Check sheet for the drawn part. Datum: minimum x, y, z corner. Units: mm. A direction names the side the tool comes from. Round coordinates to 2 decimals unless told otherwise and drop trailing zeros. Loops run counter-clockwise (first coordinate to the right, second up) from the corner with the lowest first, then second, coordinate; pieces in that order, holes last. Notation, with made-up numbers: (18.5, 16.5) -> (48.5, 16.5) arc R7 ccw to (48.5, 28.5) -> close; hole circle Ø9 at (34.5, 13). An arc over 180 degrees is marked (long way). Write item = value, one per line. Start each with the question number.
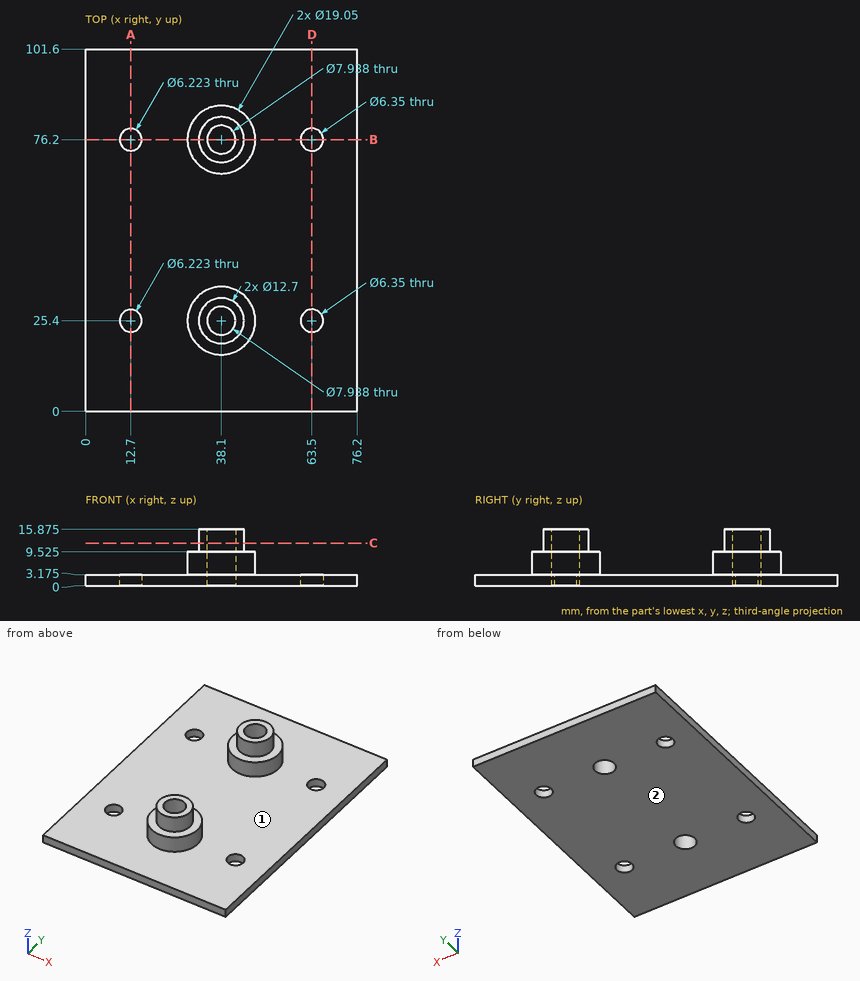
(1) Section check A-A on x = 12.7. Enter the section's corners in (y, z) (1 decimal), then the cut area to 3 significant figures.
(2) Depth check by flat-ended pin: pin 1 Ø4 at (x, y) = (51, 84) entering from +Z (1 decimal); pin 2 Ø6 at (x, z) = (41.5, 8) entering from -Y; pin 3 Ø8 at (x, z) = (31.5, 11.5) entering from -Y. Enter the tip coordinate at first touch or a pass-through.
(3) Access from +Z, -Z, +X, -X, +Y, -Y to the whole of each face (thin tool, end or side, straight path). Record for the marked faces 1 and 2.
(4) Section check C-C on z = 12. Enter the section's corners in (x, y).
(5) Section check B-B on y = 76.2. Give the number of separate pieces and of enclosed holes in the cut face.
(6) Section check D-D on x = 63.5. Enter the section's corners in (y, z) (1 decimal).
(7) Scan lines: line 1 (Y direction, x = 38, z = 9.25) (1 decimal); line 2 (Y direction, x = 63.5, z = 2.35) (1 decimal); line 3 (Z direction, x = 58, y = 71) (1 decimal). Record each from-to range of solid material in increasing order. Write a range as [from, to].
Computed values:
q1.outline = (0, 0) -> (22.3, 0) -> (22.3, 3.2) -> (0, 3.2) -> close; (28.5, 0) -> (73.1, 0) -> (73.1, 3.2) -> (28.5, 3.2) -> close; (79.3, 0) -> (101.6, 0) -> (101.6, 3.2) -> (79.3, 3.2) -> close
q1.area = 283 mm²
q2.pin_1 = 3.2
q2.pin_2 = 15.88
q2.pin_3 = 16.4
q3.face_1 = +Z
q3.face_2 = -Z, +X, -X, +Y, -Y
q4.outline = circle Ø12.7 at (38.1, 25.4); circle Ø12.7 at (38.1, 76.2); hole circle Ø7.94 at (38.1, 25.4); hole circle Ø7.94 at (38.1, 76.2)
q5.separate_pieces = 4
q5.enclosed_holes = 0
q6.outline = (0, 0) -> (22.2, 0) -> (22.2, 3.2) -> (0, 3.2) -> close; (28.6, 0) -> (73, 0) -> (73, 3.2) -> (28.6, 3.2) -> close; (79.4, 0) -> (101.6, 0) -> (101.6, 3.2) -> (79.4, 3.2) -> close
q7.line_1 = [15.9, 21.4], [29.4, 34.9], [66.7, 72.2], [80.2, 85.7]
q7.line_2 = [0, 22.2], [28.6, 73], [79.4, 101.6]
q7.line_3 = [0, 3.2]
